Source: CAD feature listing. Evaluate the final solid. Frame: model axes, mm. A direction names the side the tool comes from. Coordinates: 2 decimals unless noted, no trailing zeros. Order: outer loops, then holes, each group sorted by start corner. A loop starts at its lowest first (then second) coordinate and runs counter-clockwise, first axis right, second up.
Autodesk Fusion 360 part; units mm, degrees
sketch "Sketch1" plane through (0, 0, 0) normal (1, 0, 0) x (0, 1, 0)
  line L0 (-12.6, 18.1567) -> (7.4, 18.1567)
  line L1 (7.4, 18.1567) -> (7.4, -33.3433)
  line L2 (7.4, -33.3433) -> (1.8, -33.3433)
  line L3 (1.8, -1.5933) -> (-12.6, -1.5933)
  line L4 (-12.6, -1.5933) -> (-12.6, 18.1567)
  circle A0 centre (-2.6, 8.1567) radius 3
  line L5 (7.4, 18.1567) -> (-2.6, 8.1567) construction
  line L6 (-12.6, 18.1567) -> (-2.6, 8.1567) construction
  arc A1 (1.8, -18.5433) -> (1.8, -16.9433) centre (3.3, -17.7433) ccw
  line L7 (1.8, -33.3433) -> (1.8, -18.5433)
  line L8 (1.8, -16.9433) -> (1.8, -1.5933)
  line L9 (2.244, -16.4933) -> (1.356, -16.4933)
  line L10 (1.356, -16.4933) -> (1.356, -18.9933)
  line L11 (1.356, -18.9933) -> (2.244, -18.9933)
  line L12 (2.244, -18.9933) -> (2.244, -16.4933)
  line L13 (2.244, -16.4933) -> (1.356, -18.9933) construction
  line L14 (1.356, -16.4933) -> (2.244, -18.9933) construction
  line L15 (3.3, -17.7433) -> (-0.8, -17.7433) construction
  point P0 (1.8, -17.7433)
  dimension "d1" = 20
  dimension "d2" = 19.75
  dimension "d3" = 6
  dimension "d4" = 45
  dimension "d5" = 45
  dimension "d6" = 5.6
  dimension "d7" = 3.4
  dimension "d8" = 15.6
  dimension "d10" = 1.5
  dimension "d24" = 31.75
  dimension "d25" = 8.1567
  dimension "d26" = 2.5
extrude "Extrude1" add sketch "Sketch1" along normal mid plane 4 contours L0 L1 L2 L3 L4 A1 L7 L8 L9 L11
fillet "Fillet1" radius 4 2 edges at (0, -12.6, 18.1567) (0, 7.4, 18.1567)
fillet "Fillet2" radius 2 1 edges at (0, -12.6, -1.5933)
fillet "Fillet3" radius 3.4 1 edges at (0, 1.8, -1.5933)
fillet "Fillet4" radius 0.4 1 edges at (0, 1.8, -33.3433)
fillet "Fillet5" radius 3 1 edges at (0, 7.4, -33.3433)
chamfer "Chamfer1" distance 0.4 angle 45 28 edges at (2, -2.6, 18.1567) (2, -11.4284, 16.9851) (2, -12.6, 7.2817) (2, -12.0142, -1.0075) (2, -6.1, -1.5933) (2, 0.8042, -2.5891) (2, 1.8, -10.7433) (2, 1.8, -25.9683) (2, 1.9172, -33.2261) (2, 3.3, -33.3433) (2, 6.5213, -32.4646) (2, 7.4, -8.0933) (2, 6.2284, 16.9851) (2, -5.397, 9.2416) (-2, -2.6, 18.1567) (-2, 6.2284, 16.9851) (-2, 7.4, -8.0933) (-2, 6.5213, -32.4646) (-2, 3.3, -33.3433) (-2, 1.9172, -33.2261) (-2, 1.8, -25.9683) (-2, 1.8, -10.7433) (-2, 0.8042, -2.5891) (-2, -6.1, -1.5933) (-2, -12.0142, -1.0075) (-2, -12.6, 7.2817) (-2, -11.4284, 16.9851) (-2, -5.397, 7.0719)
Q1. Set-up query: faces 1 (the conical face through (-1.886, -11.825, -0.792)), 2 (the flat face through (0, 1.8, -26)). Return all of +Z, -Z, +X, -X, +Y, -Y with unobstructed straight access to the full face (end or side cutting, diameter ignored); none if empty.
Solutions:
face 1: -Z, -X, -Y
face 2: -Z, +X, -X, -Y
Q2. Pin query (flat end, axial travel): P1, Ø1.6, axis at x = 0.5, y = -6.5, coming from the -Z side; P2, Ø12, axis at y = -7, z = -12, coming from the +X side. Return the tip coordinate at first contact, or that it passes through.
Solutions:
P1: stops at z = -1.59
P2: passes through
Q3. Section query C-C on x = -0.9. Output: boundary loops of the cut face in (y, z), plus the area to 3 significant figures.
Solutions:
outline: (-12.6, 0.41) arc R2 ccw to (-10.6, -1.59) - (-1.6, -1.59) arc R3.4 cw to (1.8, -4.99) - (1.8, -16.49) - (2.15, -16.49) arc R1.7 cw (long way) to (2.15, -18.99) - (1.8, -18.99) - (1.8, -32.94) arc R0.4 ccw to (2.2, -33.34) - (4.4, -33.34) arc R3 ccw to (7.4, -30.34) - (7.4, 14.16) arc R4 ccw to (3.4, 18.16) - (-8.6, 18.16) arc R4 ccw to (-12.6, 14.16) - close; hole circle Ø6 at (-2.6, 8.16)
area: 528 mm2
Q4. Material intervals for line 1 along Z through (x, y) = (-0.2, -2.6); line 2 along Z through (x, y) = (-0.65, 3.3); line 3 along Z through (x, y) = (-0.7, -6.5), sorted ascending.
Solutions:
line 1: z = -1.59 to 5.16, 11.16 to 18.16
line 2: z = -33.34 to -19.44, -16.04 to 18.16
line 3: z = -1.59 to 18.16
Q5. Section query B-B on z = -27.5. Output: boundary loops of the cut face in (x, y), plus the area to 3 significant figures.
Solutions:
outline: (-2, 2.2) - (-1.6, 1.8) - (1.6, 1.8) - (2, 2.2) - (2, 7) - (1.6, 7.4) - (-1.6, 7.4) - (-2, 7) - close
area: 22.1 mm2
Q6. Section query A-A on y = -2.6. Output: boundary loops of the cut face in (x, z), plus the area to 3 significant figures.
Solutions:
outline: (-2, -1.19) - (-1.6, -1.59) - (1.6, -1.59) - (2, -1.19) - (2, 4.76) - (1.6, 5.16) - (-1.6, 5.16) - (-2, 4.76) - close; (-2, 11.56) - (-1.6, 11.16) - (1.6, 11.16) - (2, 11.56) - (2, 17.76) - (1.6, 18.16) - (-1.6, 18.16) - (-2, 17.76) - close
area: 54.4 mm2
Q7. Section query D-D on z = -18. Output: boundary loops of the cut face in (x, y).
Solutions:
outline: (-2, 4.98) - (2, 4.98) - (2, 7) - (1.6, 7.4) - (-1.6, 7.4) - (-2, 7) - close
